Autodesk Inventor part; units mm, degrees
ref_plane "作業平面1" through (-29.5, -40, 30.5) normal (0, 0, -1) x (0, 1, 0)
ref_plane "YZ Plane" through (0, 0, 0) normal (1, 0, 0) x (0, 1, 0)
ref_plane "XZ Plane" through (0, 0, 0) normal (0, 1, 0) x (-1, 0, 0)
sketch "スケッチ1" plane through (0, 0, 0) normal (0, 0, 1) x (1, 0, 0)
  circle A0 centre (-7.5, 32.5) radius 1.6
  circle A1 centre (7.5, -32.5) radius 1.6
  circle A2 centre (7.5, 32.5) radius 1.6
  circle A3 centre (-7.5, -32.5) radius 1.6
  circle A4 centre (15.5, 0) radius 1.1
  circle A5 centre (10.5, -5) radius 1.1
  circle A6 centre (5.5, 0) radius 1.1
  circle A7 centre (10.5, 5) radius 1.1
  arc A8 (-10.5, -38) -> (-8.5, -40) centre (-8.5, -38) ccw
  line L0 (-8.5, -40) -> (8.5, -40)
  arc A9 (8.5, -40) -> (10.5, -38) centre (8.5, -38) ccw
  line L1 (10.5, -38) -> (10.5, -27)
  arc A10 (12.5, -25) -> (10.5, -27) centre (12.5, -27) ccw
  line L2 (12.5, -25) -> (18.5, -25)
  arc A11 (18.5, -25) -> (20.5, -23) centre (18.5, -23) ccw
  line L3 (20.5, -23) -> (20.5, 23)
  arc A12 (20.5, 23) -> (18.5, 25) centre (18.5, 23) ccw
  line L4 (18.5, 25) -> (12.5, 25)
  arc A13 (10.5, 27) -> (12.5, 25) centre (12.5, 27) ccw
  line L5 (10.5, 27) -> (10.5, 38)
  arc A14 (10.5, 38) -> (8.5, 40) centre (8.5, 38) ccw
  line L6 (8.5, 40) -> (-8.5, 40)
  arc A15 (-8.5, 40) -> (-10.5, 38) centre (-8.5, 38) ccw
  line L7 (-10.5, 38) -> (-10.5, 27)
  arc A16 (-12.5, 25) -> (-10.5, 27) centre (-12.5, 27) ccw
  line L8 (-12.5, 25) -> (-27.5, 25)
  arc A17 (-27.5, 25) -> (-29.5, 23) centre (-27.5, 23) ccw
  line L9 (-29.5, 23) -> (-29.5, -23)
  arc A18 (-29.5, -23) -> (-27.5, -25) centre (-27.5, -23) ccw
  line L10 (-27.5, -25) -> (-12.5, -25)
  arc A19 (-10.5, -27) -> (-12.5, -25) centre (-12.5, -27) ccw
  line L11 (-10.5, -27) -> (-10.5, -38)
  circle A20 centre (-8, 38) radius 1.1
  circle A21 centre (-8, -38) radius 1.1
  circle A22 centre (8, -38) radius 1.1
  circle A23 centre (8, 38) radius 1.1
  circle A24 centre (7.5, -32.5) radius 3
  circle A25 centre (7.5, 32.5) radius 3
  line L12 (12.5, 22) -> (17.5, 22)
  line L13 (17.5, 22) -> (17.5, -22)
  line L14 (17.5, -22) -> (12.5, -22)
  arc A26 (12.5, -22) -> (7.5, -27) centre (12.5, -27) ccw
  line L15 (7.5, -27) -> (7.5, -37)
  line L16 (7.5, -37) -> (-7.5, -37)
  line L17 (-7.5, -37) -> (-7.5, -27)
  arc A27 (-7.5, -27) -> (-12.5, -22) centre (-12.5, -27) ccw
  line L18 (-12.5, -22) -> (-26.5, -22)
  line L19 (-26.5, -22) -> (-26.5, 22)
  line L20 (-26.5, 22) -> (-12.5, 22)
  arc A28 (-12.5, 22) -> (-7.5, 27) centre (-12.5, 27) ccw
  line L21 (-7.5, 27) -> (-7.5, 37)
  line L22 (-7.5, 37) -> (7.5, 37)
  line L23 (7.5, 37) -> (7.5, 27)
  arc A29 (7.5, 27) -> (12.5, 22) centre (12.5, 27) ccw
  circle A30 centre (7.5, -32.5) radius 1.3
  circle A31 centre (7.5, 32.5) radius 1.3
  point P0 (0, 0)
  point P1 (7.5, -29.5)
  point P2 (10.5, -32.5)
  point P3 (10.5, 32.5)
  point P4 (7.5, 29.5)
  point P5 (17.5, 0.4583)
  point P6 (17.5, -0.4583)
  point P7 (7.5, -33.8)
  point P8 (7.5, -31.2)
  point P9 (7.5, -30.9)
  point P10 (7.5, -34.1)
  point P11 (7.5, 35.5)
  point P12 (7.5, -35.5)
  dimension "d0" = 6
  dimension "d1" = 6
  dimension "d2" = 3
  dimension "d5" = 2.6
  dimension "d6" = 2.6
ref_plane "作業平面1" through (-29.5, -40, 30.5) normal (0, 0, -1) x (0, 1, 0)
extrude "押し出し1" add sketch "スケッチ1" along normal up to surface (30.5 mm away) contours L23 A2 A25 | A25 L23 A2 | L5 A13 L4 A12 L3 A11 L2 A10 L1 A24 L15 A26 L14 L13 L12 A29 L23 A25 | L23 A31 A2 | A2 L23 A31 | A31 L23 | L23 A31 | L15 A1 A24 | A24 L15 A1 | L15 A30 A1 | A1 L15 A30
properties part number "mune_1" material "ABS プラスチック"
Geometry: final body of the model. Coordinates: model frame, mm. A direction names the side the tool comes from. Round coordinates to 2 decimals unless told otherwise and drop trailing zeros. Order: outer loops, then holes, each group sorted by start corner. A loop starts at its lowest first (then second) coordinate and runs counter-clockwise, first axis right, second up. Notation, with made-up numbers: (25, 4.5) - (33, 4.5) arc R30 ccw to (33, 40.5) - close; hole circle Ø5 at (64, 77.25). An arc over 180 degrees is marked (long way). Use CSV: the item, a comma, the result in double quotes. Start each with the question number.
Q1. Mould query, pull axis Y, two halves, no side actions, for faces 1 (the face through (19.93, -24.4, 15.04)), 2 (the face through (19.9, 24.43, 15.04)), 3 (the face through (5.45, -34.69, 15.04)). Classes: +Y half, -Y half, draft (parallel to the pull), parting line (faces both ways), or undercut.
Q2. Section query A-A (z = 20.5). Return loops of the section in (x, y).
Q3. Access query for faces 4 (the face through (15, -25, 15)), 5 (the face through (10.5, 30, 15)), 6 (the face through (15, 22, 15)). Directions: +Z, -Z, +X, -X, +Y, -Y. A direction counts if a zero-diameter tool reaches every point of the face in a straight line with its end or side. Return the directions, or none.
Q4. Material intervals for line 1 along X through (y, z) = (-32.5, 12); line 2 along Y through (x, z) = (17.25, 13.5); line 3 along X through (y, z) = (-2.5, 12.5), sorted ascending. Write a range as from..to.
Q5. Section query B-B (x = 9.75). Return loops of the section in (y, z), and give its area (3 significant figures).
Q6. Section query C-C (y = 12). Return loops of the section in (x, z).
Q7. First-contact query: pin 1 (0.8 mm diameter, centred on y = -28.5, z = 20, fed in from -X); pin 2 (4 mm diameter, centred on x = 15, z = 11, fed in from +Y); pin 3 (5 mm diameter, centred on y = -5.5, z = 21.5, fed in from -X). Flat tips, straight axial feed; report the tip coordinate or a pass-through.
Result set:
1,face 1,"-Y half"
1,face 2,"+Y half"
1,face 3,"undercut"
2,outline,"(7.5, -29.5) arc R3 ccw (long way) to (10.5, -32.5) - (10.5, -27) arc R2 cw to (12.5, -25) - (18.5, -25) arc R2 ccw to (20.5, -23) - (20.5, 23) arc R2 ccw to (18.5, 25) - (12.5, 25) arc R2 cw to (10.5, 27) - (10.5, 32.5) arc R3 ccw (long way) to (7.5, 29.5) - (7.5, 27) arc R5 ccw to (12.5, 22) - (17.5, 22) - (17.5, -22) - (12.5, -22) arc R5 ccw to (7.5, -27) - close; hole circle Ø2.6 at (7.5, -32.5)"
3,face 4,"+Z, -Z, +X, -Y"
3,face 5,"+Z, -Z, +X, +Y"
3,face 6,"+Z, -Z, -X"
4,line 1,"x = 4.5..6.2, 8.8..10.5"
4,line 2,"y = -25..-22, 22..25"
4,line 3,"x = 17.5..20.5"
5,outline,"(-34.48, 0) - (-22.82, 0) - (-22.82, 30.5) - (-34.48, 30.5) - close; (22.82, 0) - (34.48, 0) - (34.48, 30.5) - (22.82, 30.5) - close"
5,area,"711 mm2"
6,outline,"(17.5, 0) - (20.5, 0) - (20.5, 30.5) - (17.5, 30.5) - close"
7,pin 1,"stops at x = 7.5"
7,pin 2,"stops at y = 25"
7,pin 3,"stops at x = 17.5"
